```python
from build123d import *

# Parameters (mm, degrees)
SKETCH1_R           = 52.5
SKETCH1_R_2         = 50
BOSS_EXTRUDE1_DEPTH = 7.5
BOSS_EXTRUDE2_START = 2.5
SKETCH2_R           = 52.5
BOSS_EXTRUDE2_DEPTH = 2.5
SKETCH3_R           = 7.25
CUT_EXTRUDE1_DEPTH  = 75.916620319
SKETCH4_R           = 1.75
BOSS_EXTRUDE3_DEPTH = 10
FILLET1_R           = 5


with BuildPart() as part:
    # Sketch1 → Boss-Extrude1 (new body)
    with BuildSketch(Plane(origin=(0, 0, 0), x_dir=(1, 0, 0), z_dir=(0, 1, 0))):
        with Locations(Location((0, 0, 0), (0, 0, 270))):
            Circle(SKETCH1_R)
        with Locations(Location((0, 0, 0), (0, 0, 270))):
            Circle(SKETCH1_R_2, mode=Mode.SUBTRACT)
    extrude(amount=BOSS_EXTRUDE1_DEPTH)

    # Sketch2 → Boss-Extrude2 (add)
    with BuildSketch(Plane.XZ.offset(BOSS_EXTRUDE2_START)):
        with Locations(Location((0, 0, 0), (0, 0, 270))):
            Circle(SKETCH2_R)
    extrude(amount=-BOSS_EXTRUDE2_DEPTH)

    # Sketch3 → Cut-Extrude1 (cut, through all)
    with BuildSketch(Plane.XZ.offset(2.5)):
        with Locations(Location((20, 0, 0), (0, 0, 270))):
            Circle(SKETCH3_R)
        with Locations(Location((-20, 0, 0), (0, 0, 270))):
            Circle(SKETCH3_R)
    extrude(amount=-CUT_EXTRUDE1_DEPTH, mode=Mode.SUBTRACT)

    # Sketch4 → Boss-Extrude3 (add)
    with BuildSketch(Plane.XZ.offset(2.5)):
        with BuildLine():
            Line((-57.5, 5), (-52.261362401, 5))
            Line((-52.261362401, 5), (-51.658599185, 0))
            Line((-51.658599185, 0), (-52.261362401, -5))
            Line((-52.261362401, -5), (-57.5, -5))
            ThreePointArc((-57.5, -5), (-62.5, 0), (-57.5, 5))
        make_face()
        with Locations(Location((-57.5, 0, 0), (0, 0, 270))):
            Circle(SKETCH4_R, mode=Mode.SUBTRACT)
    boss_extrude3 = extrude(amount=-BOSS_EXTRUDE3_DEPTH)

    # Mirror1: Boss-Extrude3 across plane
    add(boss_extrude3.mirror(Plane(origin=(0, 0, 0), x_dir=(0, 0, 1), z_dir=(1, 0, 0))))

    # Fillet1
    fillet1_edges = [part.edges().sort_by_distance(p)[0] for p in [
        (-52.261362401, 2.5, 5),
        (-52.261362401, 2.5, -5),
        (52.261362401, 2.5, 5),
        (52.261362401, 2.5, -5),
    ]]
    fillet(fillet1_edges, radius=FILLET1_R)


solid = part.part
```
Check sheet for the modelled part. Datum: model origin and axes. Units: mm. A direction names the side the tool comes from. Coordinates: 2 decimals unless noted, no trailing zeros. Loops run counter-clockwise (first coordinate to the right, second up) from the corner with the lowest first, then second, coordinate; pieces in that order, holes last.
1) Gauge pin test, flat ends, axial feed: pin 1 (1 mm diameter, centred on x = 57, y = 4, fed in from +Z); pin 2 (3 mm diameter, centred on x = 32, y = 5.5, fed in from +Z); pin 3 (4 mm diameter, centred on y = 3, z = 19, fed in from -X); pin 4 (13 mm diameter, centred on x = 20, z = 0, fed in from -Y). Record the tip position at first contact, or that the pin passes through.
2) Release check for a two-part mould opening along X. For faces 1 (the face through (62.5, 2.4, -0.1)), 2 (the face through (-53.373, 2.57, -6.201)), 3 (the face through (1, 0, 1)) record: released by +X, released by -X, zero draft, split by the parting line, or undercut.
3) Material ranges on probe 1 along X at (y, z) = (-0.9, 0); probe 2 along X at (y, z) = (1.75, 0); probe 3 along Z at (x, y) = (9, -0.75), recorded low to high.
4) Sectioned sample at D-D (x = 0). Record the boundary of the cut face in (y, z), and give its area (3 significant figures).
5) Sectioned sample at B-B (z = 0). Record the boundary of the cut face in (x, y), and give its area (4 significant figures).
6) Sectioned sample at C-C (y = 3.25). Record the boundary of the cut face in (x, z), and give its area (3 significant figures).
7) Sectioned sample at A-A (x = 25). Record the boundary of the cut face in (y, z).
8) Access from +Z, -Z, +X, -X, +Y, -Y to the whole of each face (thin tool, end or side, straight path). Record for faces 4 (the face through (1.03, 2.43, 52.49)), 5 (the face through (15.02, 3.7, 47.69)).
Check sheet entries:
1. pin 1: stops at z = 5
1. pin 2: stops at z = 42.73
1. pin 3: stops at x = -49.67
1. pin 4: passes through
2. face 1: released by +X
2. face 2: released by -X
2. face 3: undercut
3. probe 1: x = -62.5 to -59.25, -55.75 to -27.25, -12.75 to 12.75, 27.25 to 55.75, 59.25 to 62.5
3. probe 2: x = -62.5 to -59.25, -55.75 to -50, 50 to 55.75, 59.25 to 62.5
3. probe 3: z = -51.72 to 51.72
4. outline: (-2.5, -52.5) - (7.5, -52.5) - (7.5, -50) - (0, -50) - (0, 50) - (7.5, 50) - (7.5, 52.5) - (-2.5, 52.5) - close
4. area: 300 mm2
5. outline: (-62.5, -2.5) - (-59.25, -2.5) - (-59.25, 7.5) - (-62.5, 7.5) - close; (-55.75, -2.5) - (-27.25, -2.5) - (-27.25, 0) - (-50, 0) - (-50, 7.5) - (-55.75, 7.5) - close; (-12.75, -2.5) - (12.75, -2.5) - (12.75, 0) - (-12.75, 0) - close; (27.25, -2.5) - (55.75, -2.5) - (55.75, 7.5) - (50, 7.5) - (50, 0) - (27.25, 0) - close; (59.25, -2.5) - (62.5, -2.5) - (62.5, 7.5) - (59.25, 7.5) - close
5. area: 357.5 mm2
6. outline: (-57.5, -5) - (-56.62, -5) arc R5 cw to (-51.7, -9.13) arc R52.5 ccw to (51.7, -9.13) arc R5 cw to (56.62, -5) - (57.5, -5) arc R5 ccw to (57.5, 5) - (56.62, 5) arc R5 cw to (51.7, 9.13) arc R52.5 ccw to (-51.7, 9.13) arc R5 cw to (-56.62, 5) - (-57.5, 5) arc R5 ccw to start; hole circle Ø3.5 at (-57.5, 0); hole circle Ø100 at (0, 0); hole circle Ø3.5 at (57.5, 0)
6. area: 981 mm2
7. outline: (-2.5, -46.17) - (7.5, -46.17) - (7.5, -43.3) - (0, -43.3) - (0, -5.25) - (-2.5, -5.25) - close; (-2.5, 5.25) - (0, 5.25) - (0, 43.3) - (7.5, 43.3) - (7.5, 46.17) - (-2.5, 46.17) - close
8. face 4: +Z, +Y, -Y
8. face 5: +Y
